```python
from build123d import *

# Parameters (mm, degrees)
SCHIZZO2_R                   = 1.6
SCHIZZO2_R_2                 = 1.525
ESTRUSIONE_ESTRUSIONE1_DEPTH = 1.5
RACCORDO1_R                  = 3
TAGLIO_ESTRUSIONE1_DEPTH     = 161.918381387
ESTRUSIONE_ESTRUSIONE2_START = -1.5
ESTRUSIONE_ESTRUSIONE2_DEPTH = 1.5
RACCORDO2_R                  = 0.8


with BuildPart() as part:
    # Schizzo2 → Estrusione-Estrusione1 (new body)
    with BuildSketch(Plane.XY):
        with BuildLine():
            Line((10.835450111, 45.456844872), (10.835450111, 104.878132603))
            Line((10.835450111, 104.878132603), (-7.726239407, 141.30749945))
            Line((-7.726239407, 141.30749945), (4.747851932, 147.663366447))
            Line((4.747851932, 147.663366447), (23.319883285, 111.213702604))
            ThreePointArc((23.319883285, 111.213702604), (31.262689996, 109.733445118), (37.064853942, 104.110791454))
            Line((37.064853942, 104.110791454), (67.357558736, 49.749549666))
            Line((67.357558736, 49.749549666), (55.128154906, 42.934736247))
            Line((55.128154906, 42.934736247), (24.835450111, 97.295978034))
            Line((24.835450111, 97.295978034), (24.835450111, 45.456844872))
            Line((24.835450111, 45.456844872), (10.835450111, 45.456844872))
        make_face()
        with Locations((17.835450111, 52.456844872)):
            Circle(SCHIZZO2_R, mode=Mode.SUBTRACT)
        with Locations((57.835450111, 52.456844872)):
            Circle(SCHIZZO2_R, mode=Mode.SUBTRACT)
        with Locations((1.688739761, 138.248387279)):
            Circle(SCHIZZO2_R_2, mode=Mode.SUBTRACT)
        with Locations((7.590616257, 126.665302465)):
            Circle(SCHIZZO2_R_2, mode=Mode.SUBTRACT)
    extrude(amount=ESTRUSIONE_ESTRUSIONE1_DEPTH)

    # Raccordo1
    raccordo1_edges = [part.edges().sort_by_distance(p)[0] for p in [
        (10.835450111, 45.456844872, 0.75),
        (10.835450111, 104.878132603, 0.75),
        (-7.726239407, 141.30749945, 0.75),
        (4.747851932, 147.663366447, 0.75),
        (23.319883285, 111.213702604, 0.75),
        (67.357558736, 49.749549666, 0.75),
        (55.128154906, 42.934736247, 0.75),
        (24.835450111, 97.295978034, 0.75),
        (24.835450111, 45.456844872, 0.75),
    ]]
    fillet(raccordo1_edges, radius=RACCORDO1_R)

    # Schizzo3 → Taglio-Estrusione1 (cut, through all)
    with BuildSketch(Plane(origin=(0, 0, 0), x_dir=(-1, 0, 0), z_dir=(0, 0, -1))):
        Polygon((-58.032865762, 58.26562082), (-47.760114135, 76.700406977), (-39.799110822, 78.660596286), align=None)
        Polygon((-45.099489196, 81.47498477), (-37.138485884, 83.435174078), (-27.576187875, 100.595028163), align=None)
        Polygon((-14.835450111, 73.513329832), (-20.835450111, 59.080649935), (-20.835450111, 80.754828538), align=None)
        Polygon((-20.736858212, 86.90531457), (-17.675265193, 99.811833972), (-14.835450111, 79.782808049), align=None)
    extrude(amount=-TAGLIO_ESTRUSIONE1_DEPTH, mode=Mode.SUBTRACT)

    # Schizzo4 → Estrusione-Estrusione2 (add)
    with BuildSketch(Plane(origin=(0, 0, 1.5), x_dir=(-1, 0, 0), z_dir=(0, 0, -1)).offset(ESTRUSIONE_ESTRUSIONE2_START)):
        with BuildLine():
            Line((5.053219834, 142.669470949), (-2.074832359, 146.301394947))
            ThreePointArc((-2.074832359, 146.301394947), (-4.363854842, 146.481544924), (-6.109823431, 144.990346874))
            Line((-6.109823431, 144.990346874), (-22.444537387, 112.93166566))
            ThreePointArc((-22.444537387, 112.93166566), (-23.528890764, 111.74881109), (-25.067773398, 111.294050255))
            ThreePointArc((-25.067773398, 111.294050255), (-32.027352671, 109.307494906), (-37.064853942, 104.110791454))
            Line((-37.064853942, 104.110791454), (-65.897241575, 52.370136202))
            ThreePointArc((-65.897241575, 52.370136202), (-66.162289717, 50.089384698), (-64.736972201, 48.289232505))
            Line((-64.736972201, 48.289232505), (-57.748741441, 44.395053408))
            ThreePointArc((-57.748741441, 44.395053408), (-55.467989937, 44.130005266), (-53.667837744, 45.555322782))
            Line((-53.667837744, 45.555322782), (-30.456036646, 87.209653102))
            ThreePointArc((-30.456036646, 87.209653102), (-27.081049556, 88.652933675), (-24.835450111, 85.749335941))
            Line((-24.835450111, 85.749335941), (-24.835450111, 48.456844872))
            ThreePointArc((-24.835450111, 48.456844872), (-23.956770454, 46.335524528), (-21.835450111, 45.456844872))
            Line((-21.835450111, 45.456844872), (-13.835450111, 45.456844872))
            ThreePointArc((-13.835450111, 45.456844872), (-11.714129767, 46.335524528), (-10.835450111, 48.456844872))
            Line((-10.835450111, 48.456844872), (-10.835450111, 104.157896326))
            ThreePointArc((-10.835450111, 104.157896326), (-10.752559872, 104.858232417), (-10.508469683, 105.519867825))
            Line((-10.508469683, 105.519867825), (6.364267908, 138.634479878))
            ThreePointArc((6.364267908, 138.634479878), (6.544417884, 140.92350236), (5.053219834, 142.669470949))
        make_face()
        with BuildLine():
            Line((-35.317796251, 103.13724668), (-64.150183885, 51.396591427))
            ThreePointArc((-64.150183885, 51.396591427), (-64.238533265, 50.636340926), (-63.763427427, 50.036290195))
            Line((-63.763427427, 50.036290195), (-56.775196666, 46.142111098))
            ThreePointArc((-56.775196666, 46.142111098), (-56.014946165, 46.053761717), (-55.414895434, 46.528867556))
            Line((-55.414895434, 46.528867556), (-32.203094336, 88.183197876))
            ThreePointArc((-32.203094336, 88.183197876), (-26.578115853, 90.588665498), (-22.835450111, 85.749335941))
            Line((-22.835450111, 85.749335941), (-22.835450111, 48.456844872))
            ThreePointArc((-22.835450111, 48.456844872), (-22.542556892, 47.749738091), (-21.835450111, 47.456844872))
            Line((-21.835450111, 47.456844872), (-13.835450111, 47.456844872))
            ThreePointArc((-13.835450111, 47.456844872), (-13.12834333, 47.749738091), (-12.835450111, 48.456844872))
            Line((-12.835450111, 48.456844872), (-12.835450111, 104.157896326))
            ThreePointArc((-12.835450111, 104.157896326), (-12.697299713, 105.325123145), (-12.290482732, 106.427848824))
            Line((-12.290482732, 106.427848824), (4.582254859, 139.542460877))
            ThreePointArc((4.582254859, 139.542460877), (4.642304851, 140.305468371), (4.145238835, 140.887457901))
            Line((4.145238835, 140.887457901), (-2.982813359, 144.519381899))
            ThreePointArc((-2.982813359, 144.519381899), (-3.745820853, 144.579431891), (-4.327810383, 144.082365875))
            Line((-4.327810383, 144.082365875), (-20.662524339, 112.02368466))
            ThreePointArc((-20.662524339, 112.02368466), (-22.469779967, 110.052260378), (-25.034584357, 109.294325652))
            ThreePointArc((-25.034584357, 109.294325652), (-30.99993802, 107.591563924), (-35.317796251, 103.13724668))
        make_face(mode=Mode.SUBTRACT)
    extrude(amount=ESTRUSIONE_ESTRUSIONE2_DEPTH)

    # Raccordo2
    raccordo2_edges = [part.edges().sort_by_distance(p)[0] for p in [
        (39.799110822, 78.660596286, 0.75),
        (58.032865762, 58.26562082, 0.75),
        (47.760114135, 76.700406977, 0.75),
        (45.099489196, 81.47498477, 0.75),
        (27.576187875, 100.595028163, 0.75),
        (37.138485884, 83.435174078, 0.75),
        (20.835450111, 80.754828538, 0.75),
        (14.835450111, 73.513329832, 0.75),
        (20.835450111, 59.080649935, 0.75),
        (14.835450111, 79.782808049, 0.75),
        (20.736858212, 86.90531457, 0.75),
        (17.675265193, 99.811833972, 0.75),
    ]]
    fillet(raccordo2_edges, radius=RACCORDO2_R)


solid = part.part
```
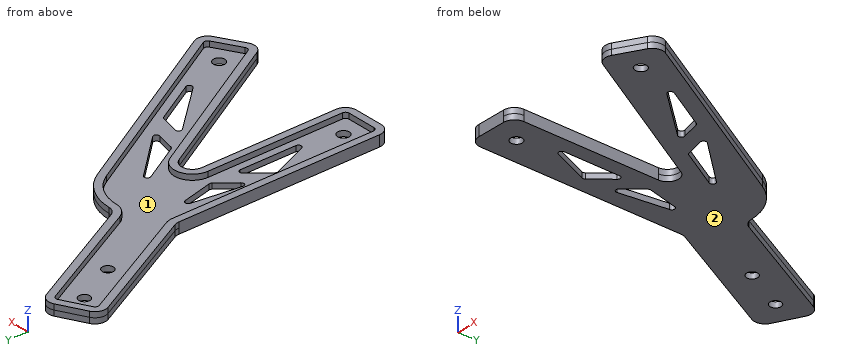
Work out the finished part from the listing and answer in its coordinate system (mm). Face numbers are marked on the shaded views. Coordinates: 2 decimals unless noted, no trailing zeros. Loops run counter-clockwise (first coordinate to the right, second up) from the corner with the lowest first, then second, coordinate; pieces in that order, holes last. Notation, with made-up numbers: (-4, -40) - (3, -40) arc R17 ccw to (3, -24) - close; hole circle Ø7 at (21.25, -30.5). An arc over 180 degrees is marked (long way). Use a Markdown table: item, result.
Item 1: The mould has two halves that part along X. Classify the marked faces 1 and 2: +X half, -X half, draft (parallel to the pull), parting line (faces both ways), or undercut.
Evaluation:
| item | result |
|---|---|
| face 1 | undercut |
| face 2 | draft |
Item 2: Find section A-A, the plane y = 59.5. Determine the outline of the cut face in (x, z).
Evaluation:
| item | result |
|---|---|
| outline | (10.84, 0) - (24.84, 0) - (24.84, 3) - (22.84, 3) - (22.84, 1.5) - (12.84, 1.5) - (12.84, 3) - (10.84, 3) - close; (45.9, 0) - (61.92, 0) - (61.92, 3) - (59.63, 3) - (59.63, 1.5) - (48.19, 1.5) - (48.19, 3) - (45.9, 3) - close |
Item 3: Find section C-C, the plane y = 92.5. Determine the outline of the cut face in (x, z).
Evaluation:
| item | result |
|---|---|
| outline | (10.84, 0) - (16.64, 0) - (16.64, 1.5) - (12.84, 1.5) - (12.84, 3) - (10.84, 3) - close; (19.41, 0) - (32.09, 0) - (32.09, 1.5) - (19.41, 1.5) - close; (35, 0) - (43.53, 0) - (43.53, 3) - (41.25, 3) - (41.25, 1.5) - (35, 1.5) - close |
Item 4: Consider probe 1 along X at (y, z) = (76, 2.55); probe 2 along X at (y, z) = (89.5, 0.35); probe 3 along X at (y, z) = (91, 1.25). Determine where each line is inside the solid, lowest interval first. Write a range as from..to.
Evaluation:
| item | result |
|---|---|
| probe 1 | x = 10.84..12.84, 22.84..24.84, 36.7..38.99, 50.44..52.73 |
| probe 2 | x = 10.84..16.21, 20.12..33.76, 37.74..45.21 |
| probe 3 | x = 10.84..16.43, 19.77..32.92, 36.37..44.37 |
Item 5: Given pin 1 Ø0.8 at (y, z) = (58, 2) entering from -X; pin 2 Ø0.8 at (y, z) = (87.5, 2.5) entering from +X; pin 3 Ø4 at (x, y) = (1.69, 138.25) entering from +Z, each flat-ended and moving along its own axis, determine where each tip first touches the part or whether it passes through.
Evaluation:
| item | result |
|---|---|
| pin 1 | stops at x = 10.84 |
| pin 2 | stops at x = 46.54 |
| pin 3 | stops at z = 1.5 |
Item 6: Find section B-B, the plane x = 34. Determine the outline of the cut face in (y, z), and give its area (3 significant figures).
Evaluation:
| item | result |
|---|---|
| outline | (80.85, 0) - (89.07, 0) - (89.07, 1.5) - (84.96, 1.5) - (84.96, 3) - (80.85, 3) - close; (93.59, 0) - (107.88, 0) - (107.88, 3) - (105.04, 3) - (105.04, 1.5) - (93.59, 1.5) - close |
| area | 44.2 mm2 |
Item 7: Find section D-D, the plane y = 124. Determine the outline of the cut face in (x, z), and give its area (3 significant figures).
Evaluation:
| item | result |
|---|---|
| outline | (1.09, 0) - (16.8, 0) - (16.8, 3) - (14.56, 3) - (14.56, 1.5) - (3.34, 1.5) - (3.34, 3) - (1.09, 3) - close |
| area | 30.3 mm2 |
